Geometry check sheet. Reference: the model listing, model coordinates, mm. A direction names the side the tool comes from. Give positions to 0.01 mm unless a question says otherwise; leave off trailing zeros. Order: outer loops, then holes, each group sorted by start corner. A loop starts at its lowest first (then second) coordinate and runs counter-clockwise, first axis right, second up. Notation, with made-up numbers: M 23.5,71 L 38.5,71 A24 cw 38.5,106 Z; hole C 56,-24.5 d8. An arc over 180 degrees is marked long. Use CSV: the item, a comma, the result in double quotes. Start each with the question number.
from build123d import *

# Parameters (mm, degrees)
SKETCH_1_R          = 1.5
EXTRUDE_1_DEPTH     = 3
SKETCH_2_W          = 15
SKETCH_2_H          = 4
CUT_EXTRUDE_1_DEPTH = 3
FILLET_1_R          = 2


with BuildPart() as part:
    # 草图1 → 凸台-拉伸1 (new body)
    with BuildSketch(Plane(origin=(0, 0, 0), x_dir=(1, 0, 0), z_dir=(0, 1, 0))):
        Polygon((-52, 0), (52, 0), (52, -17.9), (10, -17.9), (10, -10), (-10, -10), (-10, -17.9), (-52, -17.9), align=None)
        with Locations(Location((-12.5, -14.9, 0), (0, 0, 270))):
            Circle(SKETCH_1_R, mode=Mode.SUBTRACT)
        with Locations(Location((12.5, -14.9, 0), (0, 0, 90))):
            Circle(SKETCH_1_R, mode=Mode.SUBTRACT)
        with Locations(Location((-42.5, -4.9, 0), (0, 0, 270))):
            Circle(SKETCH_1_R, mode=Mode.SUBTRACT)
        with Locations(Location((42.5, -4.9, 0), (0, 0, 90))):
            Circle(SKETCH_1_R, mode=Mode.SUBTRACT)
    extrude(amount=EXTRUDE_1_DEPTH)

    # 草图2 → 切除-拉伸1 (cut)
    with BuildSketch(Plane(origin=(0, 3, 0), x_dir=(1, 0, 0), z_dir=(0, 1, 0))):
        with Locations((-25.5, -15.9)):
            Rectangle(SKETCH_2_W, SKETCH_2_H)
        with Locations((34.5, -15.9)):
            Rectangle(SKETCH_2_W, SKETCH_2_H)
    extrude(amount=-CUT_EXTRUDE_1_DEPTH, mode=Mode.SUBTRACT)

    # 圆角1
    fillet_1_edges = [part.edges().sort_by_distance(p)[0] for p in [
        (52, 1.5, 17.9),
        (10, 1.5, 17.9),
        (10, 1.5, 10),
        (-10, 1.5, 10),
        (-10, 1.5, 17.9),
        (-52, 1.5, 17.9),
        (52, 1.5, 0),
        (-52, 1.5, 0),
        (-33, 1.5, 13.9),
        (-18, 1.5, 13.9),
        (-18, 1.5, 17.9),
        (27, 1.5, 17.9),
        (27, 1.5, 13.9),
        (42, 1.5, 13.9),
        (42, 1.5, 17.9),
        (-33, 1.5, 17.9),
    ]]
    fillet(fillet_1_edges, radius=FILLET_1_R - 0.0001)  # a hair under: the kernel refuses the full size


solid = part.part
(1) Go/stop test with flat-tipped pins: P1, Ø2.5, axis at x = -42.5, z = 4.9, coming from the -Y side; P2, Ø0.9, axis at x = -23.5, y = 1, coming from the +Z side. Record where each tip stops, or that it passes through.
(2) Access from +Z, -Z, +X, -X, +Y, -Y to the whole of each face (thin tool, end or side, straight path). Record for faces 5 (the face through (-42, 1, 17.9)), 6 (the face through (42.6, 1.48, 17.33)).
(3) Sectioned sample at C-C on z = 14.9. Record the cut outline in (x, y).
(4) Draft check along Z on faces 1 (the face through (51.4, 1.52, 0.57)), 2 (the face through (-51.43, 1.52, 17.3)), 3 (the face through (-43.964, 1.479, 4.575)), 4 (the face through (-12.43, 1.48, 13.4)). Enter one of: +Z half, -Z half, draft (parallel to the pull), parting line (faces both ways), or undercut.
(5) Sectioned sample at A-A on x = -42.5. Record the cut outline in (y, z).
(6) Thickness scan on line 1 (X direction, y = 2, z = 4.9); line 2 (Z direction, x = 12.5, y = 1.7); line 3 (X direction, y = 1.6, z = 14.9). Record the ranges inside material, lowest first.
(7) Sectioned sample at B-B on z = 4.9. Record the cut outline in (x, y).
(8) Sectioned sample at D-D on y = 0.95. Give the number of separate pieces and of enclosed holes in the cut face, then the cut area to 3 significant figures.
Responses:
1,P1,"through"
1,P2,"z = 13.9"
2,face 5,"+Z, +X, -X, +Y, -Y"
2,face 6,"+Z, +Y, -Y"
3,outline,"M -52,0 L -32.73,0 L -32.73,3 L -52,3 Z; M -18.27,0 L -14,0 L -14,3 L -18.27,3 Z; M -11,0 L -10,0 L -10,3 L -11,3 Z; M 10,0 L 11,0 L 11,3 L 10,3 Z; M 14,0 L 27.27,0 L 27.27,3 L 14,3 Z; M 41.73,0 L 52,0 L 52,3 L 41.73,3 Z"
4,face 1,"-Z half"
4,face 2,"+Z half"
4,face 3,"undercut"
4,face 4,"undercut"
5,outline,"M 0,0 L 3,0 L 3,3.4 L 0,3.4 Z; M 0,6.4 L 3,6.4 L 3,17.9 L 0,17.9 Z"
6,line 1,"-52 to -44, -41 to 41, 44 to 52"
6,line 2,"0 to 13.4, 16.4 to 17.9"
6,line 3,"-52 to -32.73, -18.27 to -14, -11 to -10, 10 to 11, 14 to 27.27, 41.73 to 52"
7,outline,"M -52,0 L -44,0 L -44,3 L -52,3 Z; M -41,0 L 41,0 L 41,3 L -41,3 Z; M 44,0 L 52,0 L 52,3 L 44,3 Z"
8,separate pieces,"1"
8,enclosed holes,"4"
8,area,"1,550 mm2"
